Geometry: final body of the model. Coordinates: model frame, mm. Face numbers are marked on the shaded views. A direction names the side the tool comes from. Round coordinates to 2 decimals unless told otherwise and drop trailing zeros. Write each loop counter-clockwise with the first axis right and the second up, starting at its lowest first coordinate (ties: lowest second). Pieces come first, ordered by that corner, then holes.
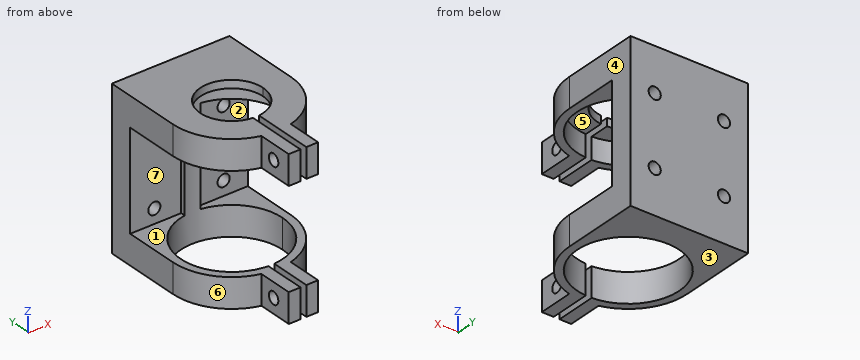
from build123d import *

# Parameters (mm, degrees)
BOSS_EXTRUDE1_DEPTH   = 20
SKETCH2_W             = 3
SKETCH2_H             = 10.5
BOSS_EXTRUDE2_DEPTH   = 20
SKETCH4_W             = 30
SKETCH4_H             = 40
BOSS_EXTRUDE3_DEPTH   = 5
SKETCH5_W             = 25
SKETCH5_H             = 37.478347352
CUT_EXTRUDE2_DEPTH    = 13
SKETCH6_R             = 1.55
MOTORMOUNTHOLES_DEPTH = 6
CLAMPHOLES_REACH      = 38.094
SKETCH8_R             = 1.55
ENDSTOPPER_DEPTH      = 2
CUT_EXTRUDE7_START    = -15
SKETCH10_W            = 25
SKETCH10_H            = 37.478347352
CUT_EXTRUDE7_DEPTH    = 13
SKETCH11_W            = 25
SKETCH11_H            = 10.633114773
CUT_EXTRUDE8_DEPTH    = 4


with BuildPart() as part:
    # Sketch1 → Boss-Extrude1 (new, symmetric)
    with BuildSketch(Plane.XY):
        with BuildLine():
            Line((-15, 15), (-15, 0))
            ThreePointArc((-15, 0), (-10.606601721, 10.606601715), (-8e-09, 15))
            Line((-8e-09, 15), (-15, 15))
        make_face()
        with BuildLine():
            Line((15, 15), (-8e-09, 15))
            ThreePointArc((-8e-09, 15), (10.606601715, 10.606601721), (15, 0))
            Line((15, 0), (15, 15))
        make_face()
        with BuildLine():
            ThreePointArc((-8e-09, 15), (-10.606601721, 10.606601715), (-15, 0))
            ThreePointArc((-15, 0), (-10.86853256, -10.338036564), (-0.75, -14.981238267))
            Line((-0.75, -14.981238267), (-0.75, -12.978347352))
            ThreePointArc((-0.75, -12.978347352), (-8.923284149, 9.453835201), (13, 0))
            ThreePointArc((13, 0), (9.453835201, -8.923284149), (0.75, -12.978347352))
            Line((0.75, -12.978347352), (0.75, -14.981238267))
            ThreePointArc((0.75, -14.981238267), (10.86853256, -10.338036564), (15, 0))
            ThreePointArc((15, 0), (10.606601715, 10.606601721), (-8e-09, 15))
        make_face()
    extrude(amount=BOSS_EXTRUDE1_DEPTH, both=True)

    # Sketch2 → Boss-Extrude2 (add, symmetric)
    with BuildSketch(Plane.XY):
        with Locations((-2.25, -18.228347352)):
            Rectangle(SKETCH2_W, SKETCH2_H)
        with Locations((2.25, -18.228347352)):
            Rectangle(SKETCH2_W, SKETCH2_H)
    extrude(amount=BOSS_EXTRUDE2_DEPTH, both=True)

    # Sketch4 → Boss-Extrude3 (add)
    with BuildSketch(Plane(origin=(0, 15, 0), x_dir=(1, 0, 0), z_dir=(0, 1, 0))):
        Rectangle(SKETCH4_W, SKETCH4_H)
    extrude(amount=BOSS_EXTRUDE3_DEPTH)

    # Sketch5 → Cut-Extrude2 (cut)
    with BuildSketch(Plane(origin=(15, 0, 0), x_dir=(0, 0, -1), z_dir=(1, 0, 0))):
        with Locations((0, -4.739173676)):
            Rectangle(SKETCH5_W, SKETCH5_H)
    extrude(amount=-CUT_EXTRUDE2_DEPTH, mode=Mode.SUBTRACT)

    # Sketch6 → MotorMountHoles (cut)
    with BuildSketch(Plane(origin=(0, 20, 0), x_dir=(1, 0, 0), z_dir=(0, 1, 0))):
        with Locations(Location((-8.838834765, 8.838834765, 0), (0, 0, 270))):
            Circle(SKETCH6_R)
        with Locations(Location((8.838834765, 8.838834765, 0), (0, 0, 270))):
            Circle(SKETCH6_R)
        with Locations(Location((8.838834765, -8.838834765, 0), (0, 0, 270))):
            Circle(SKETCH6_R)
        with Locations(Location((-8.838834765, -8.838834765, 0), (0, 0, 270))):
            Circle(SKETCH6_R)
    extrude(amount=-MOTORMOUNTHOLES_DEPTH, mode=Mode.SUBTRACT)

    # ClampHoles: up to this face of the body (flat: up to its plane)
    clampholes_end = Plane(part.part.faces().sort_by_distance((3.75, -19.00101745, 16.25))[0])
    # Sketch8 → ClampHoles (cut, up to the picked face)
    with BuildSketch(Plane.ZY.offset(3.75), mode=Mode.PRIVATE) as clampholes_sk1:
        with Locations(Location((16.25, -18.523687548, 0), (0, 0, 270))):
            Circle(SKETCH8_R)
    clampholes_tool1 = split(extrude(clampholes_sk1.sketch, amount=-CLAMPHOLES_REACH, mode=Mode.PRIVATE), bisect_by=clampholes_end, keep=Keep.BOTH, mode=Mode.PRIVATE)
    # Sketch8 → ClampHoles (cut, up to the picked face)
    with BuildSketch(Plane.ZY.offset(3.75), mode=Mode.PRIVATE) as clampholes_sk2:
        with Locations(Location((-16.25, -18.523687548, 0), (0, 0, 270))):
            Circle(SKETCH8_R)
    clampholes_tool2 = split(extrude(clampholes_sk2.sketch, amount=-CLAMPHOLES_REACH, mode=Mode.PRIVATE), bisect_by=clampholes_end, keep=Keep.BOTH, mode=Mode.PRIVATE)
    add(clampholes_tool1.solids().sort_by(Axis((-3.75, -18.523688, 16.25), (1, 0, 0)))[0], mode=Mode.SUBTRACT)
    add(clampholes_tool2.solids().sort_by(Axis((-3.75, -18.523688, -16.25), (1, 0, 0)))[0], mode=Mode.SUBTRACT)

    # Sketch9 → EndStopper (add)
    with BuildSketch(Plane.XY.offset(20)):
        with BuildLine():
            ThreePointArc((13, 0), (-8.923284149, 9.453835201), (-0.75, -12.978347352))
            Line((-0.75, -12.978347352), (-0.75, -7.964766161))
            ThreePointArc((-0.75, -7.964766161), (-5.385164807, 5.916079783), (8, 0))
            ThreePointArc((8, 0), (5.916079783, -5.385164807), (0.75, -7.964766161))
            Line((0.75, -7.964766161), (0.75, -12.978347352))
            ThreePointArc((0.75, -12.978347352), (9.453835201, -8.923284149), (13, 0))
        make_face()
    extrude(amount=-ENDSTOPPER_DEPTH)

    # Sketch10 → Cut-Extrude7 (cut)
    with BuildSketch(Plane(origin=(0, 0, 0), x_dir=(0, 0, -1), z_dir=(1, 0, 0)).offset(CUT_EXTRUDE7_START)):
        with Locations((0, -4.739173676)):
            Rectangle(SKETCH10_W, SKETCH10_H)
    extrude(amount=CUT_EXTRUDE7_DEPTH, mode=Mode.SUBTRACT)

    # Sketch11 → Cut-Extrude8 (cut)
    with BuildSketch(Plane.ZY.offset(2)):
        with Locations((0, -18.161789965)):
            Rectangle(SKETCH11_W, SKETCH11_H)
    extrude(amount=-CUT_EXTRUDE8_DEPTH, mode=Mode.SUBTRACT)


solid = part.part
1) Draft query along X for the marked faces 4, 5, 6 and 7. Return one class per face: pulls with the +X half, pulls with the -X half, needs draft (parallel to the pull), parting line crosses it, or undercut.
2) Section C-C on x = -5.25. Output: boundary loops of the cut face in (y, z), plus the area to 3 significant figures.
3) Section D-D on z = -11. Output: boundary loops of the cut face in (x, y), plus the area to 3 significant figures.
4) Line query: probe 1 along X at (y, z) = (-17, -14.5); probe 2 along Y at (x, z) = (4, 1); probe 3 along Z at (x, y) = (-0.25, 10). Output: solid intervals per line, ascending.
5) First-contact query: P1, Ø6, axis at y = -20, z = -17, coming from the -X side; P2, Ø2, axis at y = -14.5, z = 16, coming from the -X side; P3, Ø4, axis at y = -18.52, z = -16.25, coming from the +X side; P4, Ø2.5, axis at y = -18.52, z = -16.25, coming from the +X side. Flat tips, straight axial feed; report the tip coordinate or a pass-through.
6) Section B-B on x = -12. Output: boundary loops of the cut face in (y, z).
7) Section A-A on z = -16.25. Output: boundary loops of the cut face in (x, y), plus the area to 3 significant figures.
8) Reachability of the marked faces 1, 2 and 3 from +Z, -Z, +X, -X, +Y, -Y: full face, straight path, thin tool, end or side. Return the list, or none.
Filled in:
1. face 4: pulls with the +X half
1. face 5: undercut
1. face 6: pulls with the -X half
1. face 7: needs draft
2. outline: (-14.05, -20) - (-11.89, -20) - (-11.89, -12.5) - (-14.05, -12.5) - close; (-14.05, 12.5) - (-11.89, 12.5) - (-11.89, 18) - (-6.04, 18) - (-6.04, 20) - (-14.05, 20) - close; (6.04, 18) - (11.89, 18) - (11.89, 12.5) - (14, 12.5) - (14, -12.5) - (11.89, -12.5) - (11.89, -20) - (20, -20) - (20, 20) - (6.04, 20) - close
2. area: 327 mm2
3. outline: (-15, 14) - (-2, 14) - (-2, 12.85) arc R13 cw to (2, 12.85) - (2, 14) - (15, 14) - (15, 20) - (-15, 20) - close
3. area: 184 mm2
4. probe 1: x = -3.75 to -0.75, 0.75 to 3.75
4. probe 2: y = 14 to 20
4. probe 3: z = 18 to 20
5. P1: stops at x = -3.75
5. P2: stops at x = -6.54
5. P3: stops at x = 3.75
5. P4: passes through
6. outline: (-9, -20) - (-5, -20) - (-5, -12.5) - (-9, -12.5) - close; (-9, 12.5) - (-5, 12.5) - (-5, 18) - (5, 18) - (5, 12.5) - (14, 12.5) - (14, -12.5) - (5, -12.5) - (5, -20) - (20, -20) - (20, 20) - (-9, 20) - close
7. outline: (-15, 0) arc R15 ccw to (-3.75, -14.52) - (-3.75, -16.97) - (-0.75, -16.97) - (-0.75, -12.98) arc R13 cw (long way) to (0.75, -12.98) - (0.75, -16.97) - (3.75, -16.97) - (3.75, -14.52) arc R15 ccw to (15, 0) - (15, 20) - (-15, 20) - close; (-3.75, -23.48) - (-0.75, -23.48) - (-0.75, -20.07) - (-3.75, -20.07) - close; (0.75, -23.48) - (3.75, -23.48) - (3.75, -20.07) - (0.75, -20.07) - close
7. area: 453 mm2
8. face 1: -X, -Y
8. face 2: +X, -Y
8. face 3: -Z, +X, -X, +Y, -Y
